The model under review builds one solid part; all positions refer to its coordinate system, in mm. Face numbers are marked on the shaded views. Coordinates: 2 decimals unless noted, no trailing zeros. Loops run counter-clockwise (first coordinate to the right, second up) from the corner with the lowest first, then second, coordinate; pieces in that order, holes last. Notation, with made-up numbers: (85.5, 71) -> (106.5, 71) arc R24 cw to (106.5, 104) -> close; hole circle Ø5 at (-16.75, 77). An arc over 180 degrees is marked (long way). One line per question, with ' | ' between items. Start each with the question number.
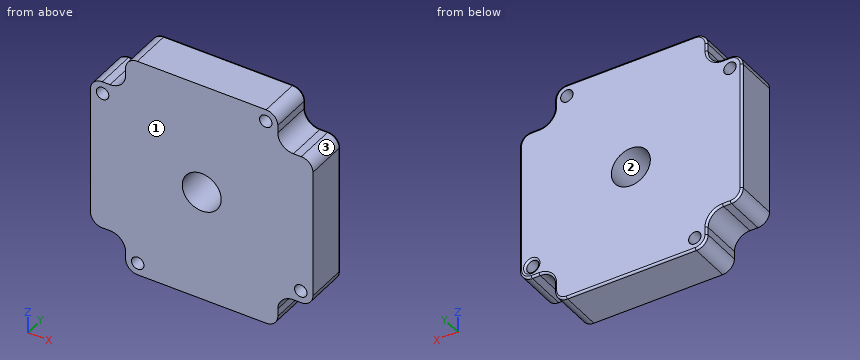
from build123d import *

# Parameters (mm, degrees)
SHAPEBINDER001_R = 1.6
PAD008_DEPTH     = 11
SKETCH014_R      = 5
POCKET007_DEPTH  = 42.001
FILLET002_R      = 0.5


with BuildPart() as part:
    # ShapeBinder001 → Pad008 (new body)
    with BuildSketch(Plane(origin=(0, 31, 0), x_dir=(1, 0, 0), z_dir=(0, 1, 0))):
        with BuildLine():
            Line((-16.5, -28.5), (16.5, -28.5))
            ThreePointArc((16.5, -28.5), (18.62132, -27.62132), (19.5, -25.5))
            Line((19.5, -25.5), (19.5, -23.5))
            ThreePointArc((19.5, -23.5), (20.671573, -20.671573), (23.5, -19.5))
            Line((23.5, -19.5), (25.5, -19.5))
            ThreePointArc((25.5, -19.5), (27.62132, -18.62132), (28.5, -16.5))
            Line((28.5, -16.5), (28.5, 16.5))
            ThreePointArc((28.5, 16.5), (27.62132, 18.62132), (25.5, 19.5))
            Line((25.5, 19.5), (23.5, 19.5))
            ThreePointArc((23.5, 19.5), (20.671573, 20.671573), (19.5, 23.5))
            Line((19.5, 23.5), (19.5, 25.5))
            ThreePointArc((19.5, 25.5), (18.62132, 27.62132), (16.5, 28.5))
            Line((16.5, 28.5), (-16.5, 28.5))
            ThreePointArc((-16.5, 28.5), (-18.62132, 27.62132), (-19.5, 25.5))
            Line((-19.5, 25.5), (-19.5, 23.5))
            ThreePointArc((-19.5, 23.5), (-20.671573, 20.671573), (-23.5, 19.5))
            Line((-23.5, 19.5), (-25.5, 19.5))
            ThreePointArc((-25.5, 19.5), (-27.62132, 18.62132), (-28.5, 16.5))
            Line((-28.5, 16.5), (-28.5, -16.5))
            ThreePointArc((-28.5, -16.5), (-27.62132, -18.62132), (-25.5, -19.5))
            Line((-25.5, -19.5), (-23.5, -19.5))
            ThreePointArc((-23.5, -19.5), (-20.671573, -20.671573), (-19.5, -23.5))
            Line((-19.5, -23.5), (-19.5, -25.5))
            ThreePointArc((-19.5, -25.5), (-18.62132, -27.62132), (-16.5, -28.5))
        make_face()
        with Locations((-16.4, 25.4)):
            Circle(SHAPEBINDER001_R, mode=Mode.SUBTRACT)
        with Locations((-25.4, -16.4)):
            Circle(SHAPEBINDER001_R, mode=Mode.SUBTRACT)
        with Locations((25.4, 16.4)):
            Circle(SHAPEBINDER001_R, mode=Mode.SUBTRACT)
        with Locations((16.4, -25.4)):
            Circle(SHAPEBINDER001_R, mode=Mode.SUBTRACT)
    extrude(amount=PAD008_DEPTH)

    # Sketch014 → Pocket007 (cut, through all)
    with BuildSketch(Plane.XZ):
        Circle(SKETCH014_R)
    extrude(amount=-POCKET007_DEPTH, mode=Mode.SUBTRACT)

    # Fillet002
    fillet002_edges = [part.edges().sort_by_distance(p)[0] for p in [
        (20.671573, 42, -20.671573),
        (25.4, 42, -14.8),
    ]]
    fillet(fillet002_edges, radius=FILLET002_R)


solid = part.part
1) Wall thickness on L1, parallel to X at y = 39, z = 25.4; L2, parallel to Z at x = -16.4, y = 34.25; L3, parallel to X at y = 39.25, z = -25.4: over which ranges is each line inside the solid? List them lowest first.
2) Insertion check: pin 1 Ø0.6 at (x, y) = (24.5, 33.5) entering from -Z; pin 2 Ø2 at (y, z) = (38, -24.5) entering from +X; pin 3 Ø3.5 at (x, z) = (25.4, -16.4) entering from -Y; pin 4 Ø2.5 at (x, z) = (16.4, 25.4) entering from +Y. Each pin has a flat end and moves straight along its axis. Give the tip position at first contact, or say it passes through.
3) Consider section C-C, the plane y = 34. Give the number of separate pieces and of enclosed holes in the cut face, plus the area to 3 significant figures.
4) Consider section B-B, the plane x = 0. Write out the cut boundary in (y, z).
5) Mouldability with a two-part tool opening along Z and no side actions: class the marked faces 1, 2 and 3 as +Z half, -Z half, draft (parallel to the pull), parting line (faces both ways), or undercut.
6) Consider section A-A, the plane z = 0. Write out the cut boundary in (x, y), plus the area to 3 significant figures.
Filled sheet:
1) L1: -19.5 to 14.8, 18 to 19.5 | L2: -28.5 to -27, -23.8 to 28.5 | L3: -19.5 to -18, -14.8 to 19.5
2) pin 1: z = -19.5 | pin 2: x = 19.5 | pin 3: y = 31 | pin 4: through
3) separate pieces: 1 | enclosed holes: 5 | area: 2,810 mm^2
4) outline: (31, -28.5) -> (41.5, -28.5) arc R0.5 ccw to (42, -28) -> (42, -5) -> (31, -5) -> close; (31, 5) -> (42, 5) -> (42, 28) arc R0.5 ccw to (41.5, 28.5) -> (31, 28.5) -> close
5) face 1: draft | face 2: undercut | face 3: +Z half
6) outline: (-28.5, 31) -> (-5, 31) -> (-5, 42) -> (-28, 42) arc R0.5 ccw to (-28.5, 41.5) -> close; (5, 31) -> (28.5, 31) -> (28.5, 41.5) arc R0.5 ccw to (28, 42) -> (5, 42) -> close | area: 517 mm^2
